```python
from build123d import *

# Parameters (mm, degrees)
F0_R     = 15
F1_DEPTH = 10
F2_R     = 3
F3_DEPTH = 25


with BuildPart() as f1:
    # F0 (on Top) → F1 (new body)
    with BuildSketch(Plane.XY):
        with BuildLine():
            Line((4.306584, 5), (-74.297338, 5))
            Line((-74.297338, 5), (-74.297338, -5))
            Line((-74.297338, -5), (4.306584, -5))
            ThreePointArc((4.306584, -5), (45.702662, 0), (4.306584, 5))
        make_face()
        with Locations((24.702662, 0)):
            Circle(F0_R, mode=Mode.SUBTRACT)
    extrude(amount=F1_DEPTH)

    # F2 (on face) → F3 (cut)
    with BuildSketch(Plane.XZ.offset(5)):
        with Locations((-64.297338, 5)):
            Circle(F2_R)
    extrude(amount=-F3_DEPTH, mode=Mode.SUBTRACT)


solid = f1.part
```
Design review of the part built by this model. Coordinates are the model's own, in mm. A direction names the side the tool comes from. Coordinates: 2 decimals unless noted, no trailing zeros. Loops run counter-clockwise (first coordinate to the right, second up) from the corner with the lowest first, then second, coordinate; pieces in that order, holes last. Notation, with made-up numbers: (-37.5, -23.5) - (-24.5, -23.5) arc R24 ccw to (-24.5, 0.5) - close; hole circle Ø9 at (23.5, 76). An arc over 180 degrees is marked (long way). Use CSV: the item, a comma, the result in double quotes. Start each with the question number.
1) Consider section A-A on z = 5. Write out the cut boundary in (x, y), then the cut area to 3 significant figures.
2) For pin 1 Ø8 at (x, y) = (-51.5, -10) entering from -Z; pin 2 Ø6 at (y, z) = (12.5, 5.5) entering from +X; pin 3 Ø5 at (x, y) = (-49, 6) entering from +Z; pin 4 Ø2 at (y, z) = (-6.5, 9) entering from +X, all flat-tipped, find the tip position at first contact; note any pin that passes through.
3) Tool access review of faces 1 (the flat face through (-34, 5, 5)), 2 (the flat face through (-74.297, 0, 5)): name each direction out of +Z, -Z, +X, -X, +Y, -Y from which nothing blocks a thin tool from reaching the whole face with its end or side.
4) Consider section D-D on x = -58.5. Write out the cut boundary in (y, z), then the cut area to 3 significant figures.
5) Wall thickness on L1, parallel to Y at x = -38.5, z = 9.5; L2, parallel to X at y = -2, z = 4; L3, parallel to Y at x = 31, z = 8.75: over which ranges is each line inside the solid? List them lowest first. Write a range as from..to.
6) Consider section C-C on y = -13. Write out the cut boundary in (x, z).
7) The part is to be moulded in two halves that separate along Y. For faces 3 (the flat face through (-36, -5, 5)), 4 (the cylindrical face through (39.01, 4.51, 4.93)), 5 (the flat face through (-10, -1, 10)), say which applies: +Y half, -Y half, draft (parallel to the pull), parting line (faces both ways), or undercut.
8) Consider section B-B on y = 0. Write out the cut boundary in (x, z), then the cut area to 3 significant figures.
Geometry says:
1,outline,"(-74.3, -5) - (-67.3, -5) - (-67.3, 5) - (-74.3, 5) - close; (-61.3, -5) - (4.31, -5) arc R21 ccw (long way) to (4.31, 5) - (-61.3, 5) - close; hole circle Ø30 at (24.7, 0)"
1,area,"1,400 mm^2"
2,pin 1,"through"
2,pin 2,"x = 43.43"
2,pin 3,"z = 10"
2,pin 4,"x = 44.97"
3,face 1,"+Z, -Z, -X, +Y"
3,face 2,"+Z, -Z, -X, +Y, -Y"
4,outline,"(-5, 0) - (5, 0) - (5, 10) - (-5, 10) - close"
4,area,"100 mm^2"
5,L1,"-5..5"
5,L2,"-74.3..-67.13, -61.47..9.84, 39.57..45.61"
5,L3,"-20.03..-13.61, 13.61..20.03"
6,outline,"(8.21, 0) - (17.22, 0) - (17.22, 10) - (8.21, 10) - close; (32.19, 0) - (41.2, 0) - (41.2, 10) - (32.19, 10) - close"
7,face 3,"-Y half"
7,face 4,"undercut"
7,face 5,"draft"
8,outline,"(-74.3, 0) - (9.7, 0) - (9.7, 10) - (-74.3, 10) - close; (39.7, 0) - (45.7, 0) - (45.7, 10) - (39.7, 10) - close; hole circle Ø6 at (-64.3, 5)"
8,area,"872 mm^2"
